Read the model definition and answer for the solid it produces. Units are mm, in the model's axes. A direction names the side the tool comes from. Round coordinates to 2 decimals unless told otherwise and drop trailing zeros. Write each loop counter-clockwise with the first axis right and the second up, starting at its lowest first coordinate (ties: lowest second). Pieces come first, ordered by that corner, then holes. Notation, with made-up numbers: (-33.5, 7) -> (24.5, 7) arc R15 ccw to (24.5, 12) -> close; hole circle Ø7 at (-7.75, -15.75). An arc over 180 degrees is marked (long way). Return JSON: item names as keys, results as strings.
from build123d import *

# Parameters (mm, degrees)
SKETCH_1_W          = 56.4
SKETCH_1_H          = 56.4
SKETCH_1_R          = 2.55
EXTRUDE_1_DEPTH     = 96
CUT_EXTRUDE_START   = -91
SKETCH_2_W          = 9.63
SKETCH_2_H          = 9.63
SKETCH_2_R          = 2.55
SKETCH_2_W_2        = 10
SKETCH_2_H_2        = 10
CUT_EXTRUDE_1_DEPTH = 91
SKETCH_3_R          = 4
EXTRUDE_2_DEPTH     = 21
SKETCH_4_R          = 19.05
EXTRUDE_3_DEPTH     = 1.6


with BuildPart() as part:
    # 草图1 → 凸台-拉伸1 (new body)
    with BuildSketch(Plane.XY):
        Rectangle(SKETCH_1_W, SKETCH_1_H)
        with Locations((23.57, 23.57)):
            Circle(SKETCH_1_R, mode=Mode.SUBTRACT)
        with Locations((23.57, -23.57)):
            Circle(SKETCH_1_R, mode=Mode.SUBTRACT)
        with Locations((-23.57, -23.57)):
            Circle(SKETCH_1_R, mode=Mode.SUBTRACT)
        with Locations((-23.57, 23.57)):
            Circle(SKETCH_1_R, mode=Mode.SUBTRACT)
    extrude(amount=EXTRUDE_1_DEPTH)

    # 草图2 → 切除-拉伸1 (cut)
    # profile 1 of 4: a face of its own
    with BuildSketch(Plane.XY.offset(96).offset(CUT_EXTRUDE_START)):
        with Locations((-23.385, -23.385)):
            Rectangle(SKETCH_2_W, SKETCH_2_H)
        with Locations((-23.57, -23.57)):
            Circle(SKETCH_2_R, mode=Mode.SUBTRACT)
    # profile 2 of 4: a face of its own
    with BuildSketch(Plane.XY.offset(96).offset(CUT_EXTRUDE_START)):
        with Locations((23.385, -23.385)):
            Rectangle(SKETCH_2_W, SKETCH_2_H)
        with Locations((23.57, -23.57)):
            Circle(SKETCH_2_R, mode=Mode.SUBTRACT)
    # profile 3 of 4: a face of its own
    with BuildSketch(Plane.XY.offset(96).offset(CUT_EXTRUDE_START)):
        with Locations((23.385, 23.385)):
            Rectangle(SKETCH_2_W, SKETCH_2_H)
        with Locations((23.57, 23.57)):
            Circle(SKETCH_2_R, mode=Mode.SUBTRACT)
    # profile 4 of 4: a face of its own
    with BuildSketch(Plane.XY.offset(96).offset(CUT_EXTRUDE_START)):
        with Locations((-23.57, 23.57)):
            Rectangle(SKETCH_2_W_2, SKETCH_2_H_2)
    extrude(amount=CUT_EXTRUDE_1_DEPTH, mode=Mode.SUBTRACT)

    # 草图3 → 凸台-拉伸2 (add)
    with BuildSketch(Plane(origin=(0, 0, 0), x_dir=(-1, 0, 0), z_dir=(0, 0, -1))):
        with Locations(Location((0, 0, 0), (0, 0, 180))):
            Circle(SKETCH_3_R)
    extrude(amount=EXTRUDE_2_DEPTH)

    # 草图4 → 凸台-拉伸3 (add)
    with BuildSketch(Plane(origin=(0, 0, 0), x_dir=(-1, 0, 0), z_dir=(0, 0, -1))):
        with Locations(Location((0, 0, 0), (0, 0, 180))):
            Circle(SKETCH_4_R)
    extrude(amount=EXTRUDE_3_DEPTH)


solid = part.part
Item 1: Section C-C (z = 89) is taken. Give the vertices of the cut face in (x, y).
Worked answers:
{"outline": "(-28.2, -18.57) -> (-18.57, -18.57) -> (-18.57, -28.2) -> (18.57, -28.2) -> (18.57, -18.57) -> (28.2, -18.57) -> (28.2, 18.57) -> (18.57, 18.57) -> (18.57, 28.2) -> (-18.57, 28.2) -> (-18.57, 18.57) -> (-28.2, 18.57) -> close"}
Item 2: For a pull along Y with two mould halves and no side action, classify faces 4 (the flat face through (-28.2, 0, 47)), 5 (the cylindrical face through (-21.214, -24.547, 2.465)), 6 (the flat face through (-23, 18.57, 50)) as released by +Y, released by -Y, zero draft, split by the parting line, or undercut.
Worked answers:
{"face 4": "zero draft", "face 5": "undercut", "face 6": "released by +Y"}
Item 3: Flat-ended cylindrical pins translate along their axes: pin 1 (7.5 mm diameter, centred on x = 24, y = 22.5, fed in from +Z); pin 2 (3 mm diameter, centred on x = -13.5, y = -17.5, fed in from -Z); pin 3 (3 mm diameter, centred on x = -0.5, y = 8, fed in from -Z). Find the tip coordinate at first contact, or state that the pin passes through.
Worked answers:
{"pin 1": "stops at z = 5", "pin 2": "stops at z = 0", "pin 3": "stops at z = -1.6"}
Item 4: A tool of negligible diameter and unlimited length cuts with its end or side. For faces 1 (the flat face through (23, -18.57, 50)), 2 (the cylindrical face through (-4.13, 18.597, -0.789)), 3 (the flat face through (-22, 21, 5)), from which of +Z, -Z, +X, -X, +Y, -Y can it reach the whole face along a straight path? Write none if from no direction.
Worked answers:
{"face 1": "+Z, +X, -Y", "face 2": "-Z", "face 3": "+Z, -X, +Y"}
Item 5: Section A-A (x = -23.57) is taken. Give the vertices of the cut face in (y, z).
Worked answers:
{"outline": "(-28.2, 0) -> (-26.12, 0) -> (-26.12, 5) -> (-28.2, 5) -> close; (-21.02, 0) -> (21.02, 0) -> (21.02, 5) -> (18.57, 5) -> (18.57, 96) -> (-18.57, 96) -> (-18.57, 5) -> (-21.02, 5) -> close; (26.12, 0) -> (28.2, 0) -> (28.2, 5) -> (26.12, 5) -> close"}
Item 6: Section D-D (x = 0) is taken. Give the vertices of the cut face in (y, z), then the cut area to 3 significant figures.
Worked answers:
{"outline": "(-28.2, 0) -> (-19.05, 0) -> (-19.05, -1.6) -> (-4, -1.6) -> (-4, -21) -> (4, -21) -> (4, -1.6) -> (19.05, -1.6) -> (19.05, 0) -> (28.2, 0) -> (28.2, 96) -> (-28.2, 96) -> close", "area": "5,630 mm2"}
Item 7: Straight lines are drawn through the part: L1, parallel to Y at x = -23.57, z = 3.05; L2, parallel to Z at x = -18, y = -19.5; L3, parallel to Y at x = -26, z = 34. For each, find the intervals that lie inside material, in ascending order. Write a range as [from, to].
Worked answers:
{"L1": "y = [-28.2, -26.12], [-21.02, 21.02], [26.12, 28.2]", "L2": "z = [0, 96]", "L3": "y = [-18.57, 18.57]"}
